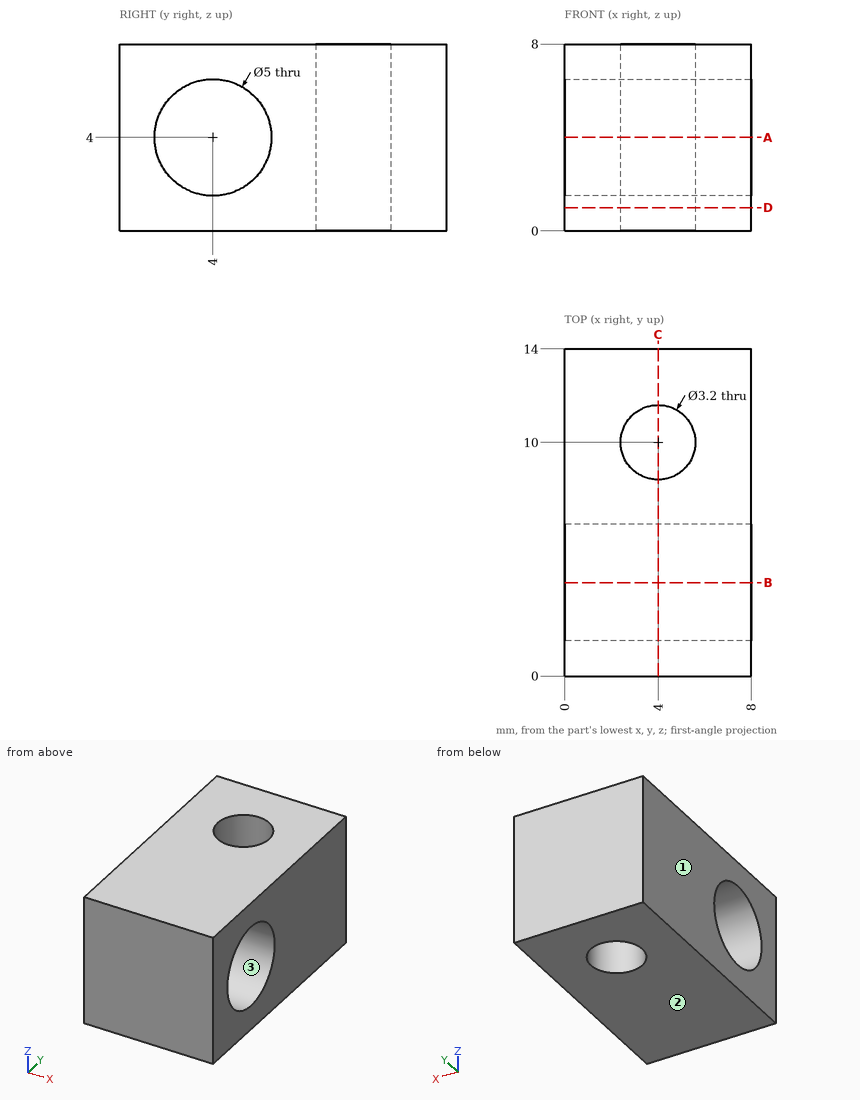
Check sheet for the drawn part. Datum: minimum x, y, z corner. Units: mm. Give positions to 0.01 mm unless a question says otherwise; leave off trailing zeros. Order: outer loops, then holes, each group sorted by start corner. A loop starts at its lowest first (then second) coordinate and runs counter-clockwise, first axis right, second up. Notation, with made-up numbers: (44.5, 20) -> (89.5, 20) arc R24 ccw to (89.5, 31) -> close; hole circle Ø3 at (22.25, -24). An arc over 180 degrees is marked (long way). Use a Markdown table: item, result.
1) Section check B-B, the plane y = 4. Record the boundary of the cut face in (x, z), then the cut area to 3 significant figures.
Results:
| item | result |
|---|---|
| outline | (0, 0) -> (8, 0) -> (8, 1.5) -> (0, 1.5) -> close; (0, 6.5) -> (8, 6.5) -> (8, 8) -> (0, 8) -> close |
| area | 24.0 mm² |
2) Section check A-A, the plane z = 4. Record the boundary of the cut face in (x, y).
Results:
| item | result |
|---|---|
| outline | (0, 0) -> (8, 0) -> (8, 1.5) -> (0, 1.5) -> close; (0, 6.5) -> (8, 6.5) -> (8, 14) -> (0, 14) -> close; hole circle Ø3.2 at (4, 10) |
3) Material ranges on probe 1 along Y at (x, z) = (3.75, 4); probe 2 along Y at (x, z) = (4, 6); probe 3 along Y at (x, z) = (6, 4), recorded low to high.
Results:
| item | result |
|---|---|
| probe 1 | 0 to 1.5, 6.5 to 8.42, 11.58 to 14 |
| probe 2 | 0 to 2.5, 5.5 to 8.4, 11.6 to 14 |
| probe 3 | 0 to 1.5, 6.5 to 14 |
4) Section check D-D, the plane z = 1. Record the boundary of the cut face in (x, y), then the cut area to 3 significant figures.
Results:
| item | result |
|---|---|
| outline | (0, 0) -> (8, 0) -> (8, 14) -> (0, 14) -> close; hole circle Ø3.2 at (4, 10) |
| area | 104 mm² |
5) Section check C-C, the plane x = 4. Record the boundary of the cut face in (y, z).
Results:
| item | result |
|---|---|
| outline | (0, 0) -> (8.4, 0) -> (8.4, 8) -> (0, 8) -> close; (11.6, 0) -> (14, 0) -> (14, 8) -> (11.6, 8) -> close; hole circle Ø5 at (4, 4) |
6) Mould release check, pull along Z, two halves, no side actions. Record for the marked faces 1, 2 and 3: pulls with the +Z half, pulls with the -Z half, needs draft (parallel to the pull), parting line crosses it, or undercut.
Results:
| item | result |
|---|---|
| face 1 | needs draft |
| face 2 | pulls with the -Z half |
| face 3 | undercut |
